Design review of the part shown in the three views and the two pictorial views. Dimensions are in mm from the part's minimum x, y and z. A direction names the side the tool comes from. Round coordinates to 2 decimals unless told otherwise and drop trailing zeros. Order: outer loops, then holes, each group sorted by start corner. A loop starts at its lowest first (then second) coordinate and runs counter-clockwise, first axis right, second up. Notation, with made-up numbers: (84, -16) - (121, -16) arc R26 ccw to (121, 11) - close; hole circle Ø2 at (5, -33.75). An arc over 180 degrees is marked (long way). One line per question, with ' | ' between items. Start each with the question number.
Item 1: Add section B-B on z = 21. State the section outline as (x, y) points.
Item 2: Add section A-A on x = 21. State the section outline as (y, z) points.
Item 3: Tool access review of the marked faces 4 and 5: name each direction out of +Z, -Z, +X, -X, +Y, -Y from which nothing blocks a thin tool from reaching the whole face with its end or side.
Item 4: For L1, parallel to X at y = 14.2, z = 21; L2, parallel to Z at x = 21, y = 6.25, list the stretches that pass through material, from the lowest coordinate up. Write a range as [from, to].
Item 5: Draft analysis for pull direction X (two halves, no side actions). For the marked faces 1, 2 and 3, state which applies: +X half, -X half, draft (parallel to the pull), parting line (faces both ways), or undercut.
Item 6: Add section C-C on y = 11.5. State the section outline as (x, z) points.
Item 7: Add section D-D on x = 33. State the section outline as (y, z) points.
Item 8: Insertion check: pin 1 Ø8 at (x, y) = (15.5, 2.5) entering from -Z; pin 2 Ø2 at (y, z) = (4.5, 6) entering from +X; pin 3 Ø2 at (y, z) = (7.5, 16.5) entering from +X. Each pin has a flat end and moves straight along its axis. Give the tip position at first contact, or say it passes through.
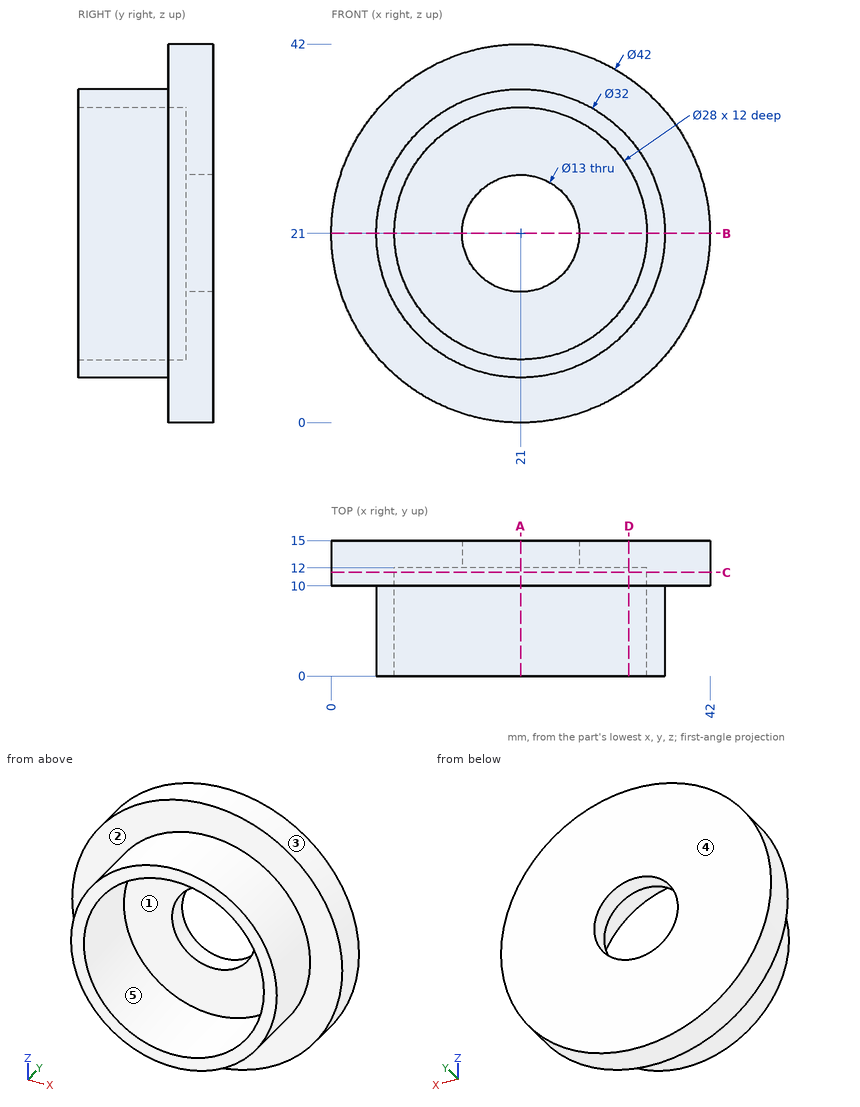
Determined:
1) outline: (0, 10) - (5, 10) - (5, 0) - (7, 0) - (7, 12) - (14.5, 12) - (14.5, 15) - (0, 15) - close; (27.5, 12) - (35, 12) - (35, 0) - (37, 0) - (37, 10) - (42, 10) - (42, 15) - (27.5, 15) - close
2) outline: (0, 5) - (10, 5) - (10, 0) - (15, 0) - (15, 14.5) - (12, 14.5) - (12, 7) - (0, 7) - close; (0, 35) - (12, 35) - (12, 27.5) - (15, 27.5) - (15, 42) - (10, 42) - (10, 37) - (0, 37) - close
3) face 4: +Z, -Z, +X, -X, +Y | face 5: -Y
4) L1: [0, 14.5], [27.5, 42] | L2: [5, 7], [35, 37]
5) face 1: undercut | face 2: draft | face 3: parting line
6) outline: circle Ø42 at (21, 21); hole circle Ø28 at (21, 21)
7) outline: (0, 10.42) - (10, 10.42) - (10, 3.77) - (15, 3.77) - (15, 38.23) - (10, 38.23) - (10, 31.58) - (0, 31.58) - (0, 28.21) - (12, 28.21) - (12, 13.79) - (0, 13.79) - close
8) pin 1: z = 5.07 | pin 2: x = 28.75 | pin 3: x = 36.61
